Read the model definition and answer for the solid it produces. Units are mm, in the model's axes. A direction names the side the tool comes from. Give positions to 0.01 mm unless a question says otherwise; leave off trailing zeros. Write each loop counter-clockwise with the first axis right and the second up, starting at its lowest first coordinate (ties: lowest second). Pieces come first, ordered by that corner, then holes. Notation, with made-up numbers: M -19,-23 L 29,-23 A17 cw 29,9 Z; hole C -33.5,18 d8. An arc over 180 degrees is marked long. Use a Markdown table: item, result. Add a question column.
Item 1: A cutting plane is placed at A-A on y = 0. Determine the outline of the cut face in (x, z), then the cut area to 3 significant figures.
Item 2: A cutting plane is placed at C-C on z = 0.4. Determine the outline of the cut face in (x, y), then the cut area to 3 significant figures.
Item 3: A cutting plane is placed at D-D on y = -7. Determine the outline of the cut face in (x, z).
Item 4: Given P1, Ø0.8, axis at y = 8.5, z = 0.5, coming from the -X side; P2, Ø0.8, axis at y = -7.5, z = -0.5, coming from the +X side, each flat-ended and moving along its own axis, determine where each tip first touches the part or whether it passes through.
Item 5: For faces 5 (the flat face through (3, -6, 0)), 6 (the flat face through (-3, 6, 0)), 7 (the flat face through (-1.75, -9, 0)), determine the directions among +Z, -Z, +X, -X, +Y, -Y from which every point of the face is accessible in a straight line to the end or side of a thin tool.
Item 6: A cutting plane is placed at B-B on x = 0. Determine the outline of the cut face in (y, z), then the cut area to 3 significant figures.
Item 7: Consider probe 1 along Y at (x, z) = (0, 0.8); probe 2 along X at (y, z) = (10.25, -0.85); probe 3 along Y at (x, z) = (-3.5, 1). Determine where each line is inside the solid, lowest interval first. Write a range as [from, to].
Item 8: The mould has two halves that part along Y. Classify faces 1 (the flat face through (0, -11, 0)), 2 (the flat face through (1.75, -8, 0)), 3 (the flat face through (3, 6, 0)), 4 (the cylindrical face through (-1.5, -0.07, -0.02)): pulls with the +Y half, pulls with the -Y half, needs draft (parallel to the pull), parting line crosses it, or undercut.
Autodesk Inventor part; units mm, degrees
ref_plane "YZ Plane" through (0, 0, 0) normal (1, 0, 0) x (0, 1, 0)
ref_plane "XZ Plane" through (0, 0, 0) normal (0, 1, 0) x (-1, 0, 0)
ref_plane "XY Plane" through (0, 0, 0) normal (0, 0, 1) x (1, 0, 0)
sketch "Sketch1" plane through (0, 0, 0) normal (0, 0, 1) x (1, 0, 0)
  line L0 (-4.5, -6) -> (4.5, -6)
  line L1 (4.5, -6) -> (4.5, 6)
  line L2 (4.5, 6) -> (-4.5, 6)
  line L3 (-4.5, 6) -> (-4.5, -6)
  line L4 (-1.75, 11) -> (1.75, 11)
  line L5 (1.75, -11) -> (-1.75, -11)
  circle A0 centre (0, 0) radius 1.5
  line L6 (1.75, 11) -> (1.75, 6)
  line L7 (1.75, -6) -> (1.75, -11)
  line L8 (-1.75, -11) -> (-1.75, -6)
  line L9 (-1.75, 6) -> (-1.75, 11)
  dimension "d0" = 3
  dimension "d1" = 12
  dimension "d2" = 9
  dimension "d3" = 3.5
  dimension "d4" = 11
  dimension "d5" = 22
  dimension "d6" = 1.75
  dimension "d7" = 4.5
extrude "Extrusion1" add sketch "Sketch1" along normal mid plane 2.8
Filled in:
| question | item | result |
|---|---|---|
| 1 | outline | M -4.5,-1.4 L -1.5,-1.4 L -1.5,1.4 L -4.5,1.4 Z; M 1.5,-1.4 L 4.5,-1.4 L 4.5,1.4 L 1.5,1.4 Z |
| 1 | area | 16.8 mm² |
| 2 | outline | M -4.5,-6 L -1.75,-6 L -1.75,-11 L 1.75,-11 L 1.75,-6 L 4.5,-6 L 4.5,6 L 1.75,6 L 1.75,11 L -1.75,11 L -1.75,6 L -4.5,6 Z; hole C 0,0 d3 |
| 2 | area | 136 mm² |
| 3 | outline | M -1.75,-1.4 L 1.75,-1.4 L 1.75,1.4 L -1.75,1.4 Z |
| 4 | P1 | x = -1.75 |
| 4 | P2 | x = 1.75 |
| 5 | face 5 | +Z, -Z, +X, -Y |
| 5 | face 6 | +Z, -Z, -X, +Y |
| 5 | face 7 | +Z, -Z, -X, -Y |
| 6 | outline | M -11,-1.4 L -1.5,-1.4 L -1.5,1.4 L -11,1.4 Z; M 1.5,-1.4 L 11,-1.4 L 11,1.4 L 1.5,1.4 Z |
| 6 | area | 53.2 mm² |
| 7 | probe 1 | [-11, -1.5], [1.5, 11] |
| 7 | probe 2 | [-1.75, 1.75] |
| 7 | probe 3 | [-6, 6] |
| 8 | face 1 | pulls with the -Y half |
| 8 | face 2 | needs draft |
| 8 | face 3 | pulls with the +Y half |
| 8 | face 4 | undercut |
